Read the model definition and answer for the solid it produces. Units are mm, in the model's axes. Coordinates: 2 decimals unless noted, no trailing zeros. Write each loop counter-clockwise with the first axis right and the second up, starting at its lowest first coordinate (ties: lowest second). Pieces come first, ordered by that corner, then holes. Notation, with made-up numbers: (-21, 49.25) -> (7, 49.25) arc R33 ccw to (7, 84.25) -> close; hole circle Ø9 at (-6.75, 2.25). An arc over 180 degrees is marked (long way). One line per item, written item: value. Start each with the question number.
1. Find section B-B, the plane x = -15. Write down the section's boundary in (y, z).
2. Find section D-D, the plane z = -18.75. Write down the section's boundary in (x, y), and give its area (3 significant figures).
3. Given P1, Ø8, axis at x = -19.5, z = -8.5, coming from the +Y side; P2, Ø4, axis at y = 23, z = -12.5, coming from the +X side, each flat-ended and moving along its own axis, determine where each tip first touches the part or whether it passes through.
4. For a pull along Z with two mould halves and no side action, classify faces 1 (the flat face through (-11, 22, 0)), 2 (the flat face through (-11, 44.196, -11)), 3 (the cylindrical face through (-7.421, 46.387, -16.793)), 4 (the flat face through (-11, 22, -23.114)) as pulls with the +Z half, pulls with the -Z half, needs draft (parallel to the pull), parting line crosses it, or undercut.
5. Consider line 1 along Y through (x, z) = (-11.5, -19.5); line 2 along Z through (x, y) = (-5, 45.5); line 3 along X through (y, z) = (46, -14). Determine where each line is inside the solid, lowest interval first.
6. Find section A-A, the plane z = -13. Write down the section's boundary in (x, y), and give its area (3 significant figures).
7. Find section C-C, the plane x = -4.25. Write down the section's boundary in (y, z).
Autodesk Inventor part; units mm, degrees
ref_plane "YZ Plane" through (0, 0, 0) normal (1, 0, 0) x (0, 1, 0)
ref_plane "XZ Plane" through (0, 0, 0) normal (0, 1, 0) x (-1, 0, 0)
ref_plane "XY Plane" through (0, 0, 0) normal (0, 0, 1) x (1, 0, 0)
sketch "Sketch1" plane through (0, 0, 0) normal (0, 1, 0) x (-1, 0, 0)
  line L0 (0, 0) -> (22.098, 0)
  line L1 (22.098, 0) -> (22.098, -23.114)
  line L2 (22.098, -23.114) -> (0, -23.114)
  line L3 (0, -23.114) -> (0, 0)
  dimension "d0" = 22.098
  dimension "d1" = 23.114
extrude "Extrusion1" add sketch "Sketch1" along normal blind 44.196
sketch "Sketch2" plane through (0, 44.196, 0) normal (0, 1, 0) x (1, 0, 0)
  circle A0 centre (-6.7327, 13.6931) radius 3.175
  point P0 (0, 0)
  dimension "d4" = 6.35
extrude "Extrusion2" add sketch "Sketch2" along normal blind 4.445
properties part number "arduino_radio_volume" material "ABS Plastic"
Answer block:
1. outline: (0, -23.11) -> (44.2, -23.11) -> (44.2, 0) -> (0, 0) -> close
2. outline: (-22.1, 0) -> (0, 0) -> (0, 44.2) -> (-22.1, 44.2) -> close
2. area: 977 mm2
3. P1: stops at y = 44.2
3. P2: stops at x = 0
4. face 1: pulls with the +Z half
4. face 2: needs draft
4. face 3: parting line crosses it
4. face 4: pulls with the -Z half
5. line 1: y = 0 to 44.2
5. line 2: z = -16.35 to -11.03
5. line 3: x = -9.89 to -3.57
6. outline: (-22.1, 0) -> (0, 0) -> (0, 44.2) -> (-3.63, 44.2) -> (-3.63, 48.64) -> (-9.83, 48.64) -> (-9.83, 44.2) -> (-22.1, 44.2) -> close
6. area: 1,000 mm2
7. outline: (0, -23.11) -> (44.2, -23.11) -> (44.2, -15.67) -> (48.64, -15.67) -> (48.64, -11.71) -> (44.2, -11.71) -> (44.2, 0) -> (0, 0) -> close
